Work out the finished part from the listing and answer in its coordinate system (mm). Face numbers are marked on the shaded views. A direction names the side the tool comes from. Round coordinates to 2 decimals unless told otherwise and drop trailing zeros. Loops run counter-clockwise (first coordinate to the right, second up) from the corner with the lowest first, then second, coordinate; pieces in that order, holes last. Notation, with made-up numbers: (38, 62) -> (80, 62) arc R12 cw to (80, 78) -> close; hole circle Ø11 at (27, 24). An arc over 180 degrees is marked (long way). Write item = value, one per line. Start each with the question number.
```python
from build123d import *

# Parameters (mm, degrees)
SKETCH1_W                 = 9.525
SKETCH1_H                 = 19.05
BOSS_EXTRUDE1_DEPTH       = 14.2875
F_8_32_TAPPED_HOLE1_D     = 3.4544
F_8_32_TAPPED_HOLE1_DEPTH = 11.43
F_8_32_TAPPED_HOLE1_TIP   = 1.037806461
SKETCH4_W                 = 3.937500126
SKETCH4_H                 = 0.79375
CUT_EXTRUDE1_DEPTH        = 25.284080433
M2X0_4_TAPPED_HOLE1_D     = 1.6


with BuildPart() as part:
    # Sketch1 → Boss-Extrude1 (new body)
    with BuildSketch(Plane(origin=(0, 0, 0), x_dir=(0, 0, -1), z_dir=(1, 0, 0))):
        Rectangle(SKETCH1_W, SKETCH1_H)
    extrude(amount=-BOSS_EXTRUDE1_DEPTH)

    # #8-32 Tapped Hole1
    with Locations(Plane(origin=(0, 0, 0), x_dir=(0, 0, -1), z_dir=(1, 0, 0))):
        with Locations((0, 6.35), (0, -6.35)):
            Hole(F_8_32_TAPPED_HOLE1_D / 2, depth=F_8_32_TAPPED_HOLE1_DEPTH)
            with Locations((0, 0, -(F_8_32_TAPPED_HOLE1_DEPTH + F_8_32_TAPPED_HOLE1_TIP / 2))):  # 118° drill point
                Cone(0, F_8_32_TAPPED_HOLE1_D / 2, F_8_32_TAPPED_HOLE1_TIP, mode=Mode.SUBTRACT)

    # Sketch4 → Cut-Extrude1 (cut, through all)
    with BuildSketch(Plane(origin=(0, 9.525, 0), x_dir=(1, 0, 0), z_dir=(0, 1, 0))):
        with Locations((-12.318749937, -4.365625)):
            Rectangle(SKETCH4_W, SKETCH4_H)
    extrude(amount=-CUT_EXTRUDE1_DEPTH, mode=Mode.SUBTRACT)

    # M2x0.4 Tapped Hole1 (through all)
    with Locations(Plane.XY.offset(3.96875)):
        with Locations((-12.7, -4.764999995), (-12.7, 4.764999995)):
            Hole(M2X0_4_TAPPED_HOLE1_D / 2)


solid = part.part
```
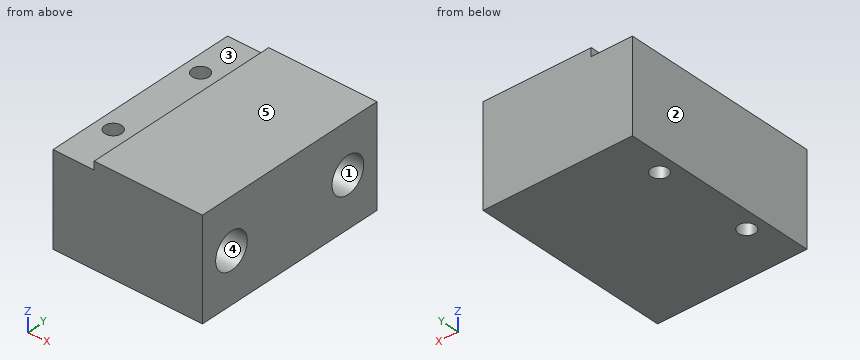
Item 1: Find the intervals of material crossed by line 1 along Y through (x, z) = (-12.7, -0.75) (3 decimals); line 2 along Y through (x, z) = (-2.25, 0) (3 decimals); line 3 along Z through (x, y) = (-8.25, 6.35), in increasing order. Write a range as [from, to].
Item 2: Section B-B (y = 4.25) is taken. Determine the outline of the cut face in (x, z), then the cut area to 3 significant figures.
Item 3: The mould has two halves that part along Z. Classify the marked faces 1, 2 and 3: pulls with the +Z half, pulls with the -Z half, needs draft (parallel to the pull), parting line crosses it, or undercut.
Item 4: Flat-ended cylindrical pins translate along their axes: pin 1 (1.2 mm diameter, centred on x = -11.5, y = 2, fed in from +Z); pin 2 (3 mm diameter, centred on y = 6.35, z = 0, fed in from +X). Find the tip coordinate at first contact, or state that the pin passes through.
Item 5: A tool of negligible diameter and unlimited length cuts with its end or side. For the marked faces 4 and 5, from which of +Z, -Z, +X, -X, +Y, -Y can it reach the whole face along a straight path? Write none if from no direction.
Item 6: Section A-A (x = -12.7) is taken. Determine the outline of the cut face in (y, z) (1 decimal).
Item 7: Section C-C (x = -3) is taken. Count the separate pieces of the cut face and the enclosed holes in it, then the cut area to 3 significant figures.
Worked answers:
q1.line_1 = [-9.525, -5.565], [-3.965, 3.965], [5.565, 9.525]
q1.line_2 = [-9.525, -8.077], [-4.623, 4.623], [8.077, 9.525]
q1.line_3 = [-4.76, -1.73], [1.73, 4.76]
q2.outline = (-14.29, -4.76) -> (-13.31, -4.76) -> (-13.31, 3.97) -> (-14.29, 3.97) -> close; (-12.09, -4.76) -> (0, -4.76) -> (0, 4.76) -> (-10.35, 4.76) -> (-10.35, 3.97) -> (-12.09, 3.97) -> close
q2.area = 122 mm2
q3.face_1 = undercut
q3.face_2 = needs draft
q3.face_3 = pulls with the +Z half
q4.pin_1 = 3.97
q4.pin_2 = -11.57
q5.face_4 = +X
q5.face_5 = +Z, +X, -X, +Y, -Y
q6.outline = (-9.5, -4.8) -> (-5.6, -4.8) -> (-5.6, 4) -> (-9.5, 4) -> close; (-4, -4.8) -> (4, -4.8) -> (4, 4) -> (-4, 4) -> close; (5.6, -4.8) -> (9.5, -4.8) -> (9.5, 4) -> (5.6, 4) -> close
q7.separate_pieces = 1
q7.enclosed_holes = 2
q7.area = 163 mm2
